```python
from build123d import *

# Parameters (mm, degrees)
BOSS_EXTRUDE1_DEPTH = 0.2
BOSS_EXTRUDE5_DEPTH = 0.435
SKETCH5_R           = 15.12
BOSS_EXTRUDE6_DEPTH = 0.01
LPATTERN1_COUNT     = 2
LPATTERN1_PITCH     = 0.4
BOSS_EXTRUDE7_DEPTH = 2.7


with BuildPart() as part:
    # Sketch1 → Boss-Extrude1 (new body)
    with BuildSketch(Plane(origin=(0, 0, 0), x_dir=(1, 0, 0), z_dir=(0, 1, 0))):
        with BuildLine():
            Line((17.249992572, 2.9475), (17.249992572, -2.9475))
            Line((17.249992572, -2.9475), (16.412681783, -6.072386409))
            ThreePointArc((16.412681783, -6.072386409), (11.243979481, -13.409807061), (3.117762689, -17.22003356))
            Line((3.117762689, -17.22003356), (-3.117762689, -17.22003356))
            ThreePointArc((-3.117762689, -17.22003356), (-11.243979481, -13.409807061), (-16.412681783, -6.072386409))
            Line((-16.412681783, -6.072386409), (-17.249992572, -2.9475))
            Line((-17.249992572, -2.9475), (-17.249992572, 2.9475))
            Line((-17.249992572, 2.9475), (-16.412681783, 6.072386409))
            ThreePointArc((-16.412681783, 6.072386409), (-12.031542367, 12.707949806), (-5.1665, 16.71996644))
            Line((-5.1665, 16.71996644), (5.1665, 16.71996644))
            ThreePointArc((5.1665, 16.71996644), (12.031542367, 12.707949806), (16.412681783, 6.072386409))
            Line((16.412681783, 6.072386409), (17.249992572, 2.9475))
        make_face()
    extrude(amount=BOSS_EXTRUDE1_DEPTH)

    # Sketch2 → Boss-Extrude5 (add)
    with BuildSketch(Plane(origin=(0, 0.2, 0), x_dir=(1, 0, 0), z_dir=(0, 1, 0))):
        with BuildLine():
            Line((-4.402806164, 16.41996644), (4.402806164, 16.41996644))
            ThreePointArc((4.402806164, 16.41996644), (11.764995572, 12.271303076), (16.22, 5.0903438))
            Line((16.22, 5.0903438), (16.22, -5.0903438))
            ThreePointArc((16.22, -5.0903438), (11.898124894, -12.142266016), (4.759884935, -16.32003356))
            Line((4.759884935, -16.32003356), (-4.759884935, -16.32003356))
            ThreePointArc((-4.759884935, -16.32003356), (-11.898124894, -12.142266016), (-16.22, -5.0903438))
            Line((-16.22, -5.0903438), (-16.22, 5.0903438))
            ThreePointArc((-16.22, 5.0903438), (-11.764995572, 12.271303076), (-4.402806164, 16.41996644))
        make_face()
    boss_extrude5 = extrude(amount=BOSS_EXTRUDE5_DEPTH)

    # Sketch5 → Boss-Extrude6 (add)
    with BuildSketch(Plane(origin=(0, 0.635, 0), x_dir=(1, 0, 0), z_dir=(0, 1, 0))):
        with Locations(Location((0, 0, 0), (0, 0, 90))):
            Circle(SKETCH5_R)
    extrude(amount=BOSS_EXTRUDE6_DEPTH)

    # LPattern1: Boss-Extrude5 ×2
    with Locations(*[(0, -i * LPATTERN1_PITCH, 0) for i in range(1, LPATTERN1_COUNT)]):
        add(boss_extrude5)

    # Sketch6 → Boss-Extrude7 (add, symmetric)
    with BuildSketch(Plane.ZY):
        with BuildLine():
            Line((17.22003356, 0.2), (18.02003356, 0.2))
            ThreePointArc((18.02003356, 0.2), (18.47003356, -0.25), (18.02003356, -0.7))
            Line((18.02003356, -0.7), (-0.77996644, -0.7))
            Line((-0.77996644, -0.7), (-0.77996644, -0.9))
            Line((-0.77996644, -0.9), (18.02003356, -0.9))
            ThreePointArc((18.02003356, -0.9), (18.67003356, -0.25), (18.02003356, 0.4))
            Line((18.02003356, 0.4), (16.77003356, 0.4))
            Line((16.77003356, 0.4), (16.77003356, 0.2))
            Line((16.77003356, 0.2), (17.22003356, 0.2))
        make_face()
    extrude(amount=BOSS_EXTRUDE7_DEPTH, both=True)


solid = part.part
```
The listing builds one solid part. Answer for the finished solid, in the listing's coordinates (mm). A direction names the side the tool comes from. Round coordinates to 2 decimals unless told otherwise and drop trailing zeros. Order: outer loops, then holes, each group sorted by start corner. A loop starts at its lowest first (then second) coordinate and runs counter-clockwise, first axis right, second up. Notation, with made-up numbers: (45.5, 56) - (68.5, 56) arc R16 ccw to (68.5, 73) - close; hole circle Ø11 at (-19, 39.25). An arc over 180 degrees is marked (long way). Put each result on its own line as item: value. Start each with the question number.
(1) Find section D-D (x = 14). Give the vertices of the cut face in (y, z) (3 decimals), plus the area to 3 significant figures.
(2) Determine the mould class of faces 1 (the flat face through (11, 0.635, 11)), 2 (the cylindrical face through (11.68, 0.41, -12.35)), 3 (the cylindrical face through (-11.814, 0.414, 12.224)), 4 (the flat face through (0, 0.2, 17.6)) for opening direction Z: released by +Z, released by -Z, zero draft, split by the parting line, or undercut.
(3) Find section C-C (z = -9.5). Give the vertices of the cut face in (x, y) (3 decimals).
(4) Straight lines are drawn through the part: probe 1 along Y at (x, z) = (0.5, 12) (3 decimals); probe 2 along Y at (x, z) = (-4.5, 10) (3 decimals); probe 3 along Z at (x, y) = (-3.5, -0.05). For each, find the intervals that lie inside material, in ascending order. Write a range as from..to.
(5) Find section B-B (x = 0). Give the vertices of the cut face in (y, z) (3 decimals).
(6) Given P1, Ø1.4, axis at x = 0, z = 17.5, coming from the +Y side; P2, Ø9.5, axis at x = 0.5, z = -8, coming from the -Y side, each flat-ended and moving along its own axis, determine where each tip first touches the part or whether it passes through.
(7) Find section A-A (z = 0). Give the vertices of the cut face in (x, y) (3 decimals).
(8) For faces 5 (the cylindrical face through (-0.04, -0.24, 18.47)), 6 (the cylindrical face through (11.98, 0.41, 12.06)), 7 (the flat face through (0, 0.4, 17)), determine the directions among +Z, -Z, +X, -X, +Y, -Y from which every point of the face is accessible in a straight line to the end or side of a thin tool.
Reply:
1. outline: (-0.2, -9.644) - (0, -9.644) - (0, -10.5) - (0.2, -10.5) - (0.2, -9.644) - (0.635, -9.644) - (0.635, -5.711) - (0.645, -5.711) - (0.645, 5.711) - (0.635, 5.711) - (0.635, 9.644) - (0.2, 9.644) - (0.2, 10.5) - (0, 10.5) - (0, 9.644) - (-0.2, 9.644) - close
1. area: 16.6 mm^2
2. face 1: zero draft
2. face 2: released by -Z
2. face 3: released by +Z
2. face 4: undercut
3. outline: (-14.697, 0) - (-14.098, 0) - (-14.098, -0.2) - (14.098, -0.2) - (14.098, 0) - (14.697, 0) - (14.697, 0.2) - (14.098, 0.2) - (14.098, 0.635) - (11.763, 0.635) - (11.763, 0.645) - (-11.763, 0.645) - (-11.763, 0.635) - (-14.098, 0.635) - (-14.098, 0.2) - (-14.697, 0.2) - close
4. probe 1: -0.9..-0.7, -0.2..0.645
4. probe 2: -0.2..0.645
4. probe 3: -16.42..16.32
5. outline: (-0.9, -0.78) - (-0.7, -0.78) - (-0.7, 18.02) arc R0.45 cw to (0.2, 18.02) - (0.2, 17.22) - (0, 17.22) - (0, 16.32) - (-0.2, 16.32) - (-0.2, -16.42) - (0, -16.42) - (0, -16.72) - (0.2, -16.72) - (0.2, -16.42) - (0.635, -16.42) - (0.635, -15.12) - (0.645, -15.12) - (0.645, 15.12) - (0.635, 15.12) - (0.635, 16.32) - (0.2, 16.32) - (0.2, 16.77) - (0.4, 16.77) - (0.4, 18.02) arc R0.65 ccw to (-0.9, 18.02) - close
6. P1: y = 0.4
6. P2: y = -0.2
7. outline: (-17.25, 0) - (-16.22, 0) - (-16.22, -0.2) - (16.22, -0.2) - (16.22, 0) - (17.25, 0) - (17.25, 0.2) - (16.22, 0.2) - (16.22, 0.635) - (15.12, 0.635) - (15.12, 0.645) - (-15.12, 0.645) - (-15.12, 0.635) - (-16.22, 0.635) - (-16.22, 0.2) - (-17.25, 0.2) - close; (-2.7, -0.9) - (2.7, -0.9) - (2.7, -0.7) - (-2.7, -0.7) - close
8. face 5: +X, -X
8. face 6: +Z, +X, +Y
8. face 7: +Z, +X, -X, +Y
